```python
from build123d import *

# Parameters (mm, degrees)
SKETCH1_W           = 10
SKETCH1_H           = 10
BOSS_EXTRUDE1_DEPTH = 205
SKETCH2_R           = 3.5
BOSS_EXTRUDE2_DEPTH = 8
SKETCH4_W           = 10
SKETCH4_H           = 10
CUT_EXTRUDE1_DEPTH  = 100


with BuildPart() as part:
    # Sketch1 → Boss-Extrude1 (new body)
    with BuildSketch(Plane.XY):
        with Locations((5, -5)):
            Rectangle(SKETCH1_W, SKETCH1_H)
    extrude(amount=BOSS_EXTRUDE1_DEPTH)

    # Sketch2 → Boss-Extrude2 (add)
    with BuildSketch(Plane(origin=(10, 0, 0), x_dir=(0, 0, -1), z_dir=(1, 0, 0))):
        with Locations((-200, -5.053950804)):
            Circle(SKETCH2_R)
    extrude(amount=BOSS_EXTRUDE2_DEPTH)

    # Sketch4 → Cut-Extrude1 (cut)
    with BuildSketch(Plane(origin=(0, 0, 0), x_dir=(-1, 0, 0), z_dir=(0, 0, -1))):
        with Locations((-5, -5)):
            Rectangle(SKETCH4_W, SKETCH4_H)
    extrude(amount=-CUT_EXTRUDE1_DEPTH, mode=Mode.SUBTRACT)


solid = part.part
```
For this review, take the finished solid that the model builds, in its own axes (mm). A direction names the side the tool comes from. Coordinates: 2 decimals unless noted, no trailing zeros. Write each loop counter-clockwise with the first axis right and the second up, starting at its lowest first coordinate (ties: lowest second). Pieces come first, ordered by that corner, then holes.
(1) For pin 1 Ø2 at (x, y) = (15, -4) entering from -Z; pin 2 Ø2 at (x, y) = (10.5, -7.5) entering from +Z; pin 3 Ø10 at (x, z) = (15.5, 158) entering from -Y, all flat-tipped, find the tip position at first contact; note any pin that passes through.
(2) Tool access review of faces 1 (the face through (18, -5, 200)), 2 (the face through (13.944, -4.003, 196.662)): name each direction out of +Z, -Z, +X, -X, +Y, -Y from which nothing blocks a thin tool from reaching the whole face with its end or side.
(3) Add section B-B on y = -7. Give the boundary of the cut face in (x, z), then the cut area to 3 significant figures.
(4) Wall thickness on probe 1 along X at (y, z) = (-1, 178); probe 2 along Z at (x, y) = (10.25, -5.25); probe 3 along Z at (x, y) = (11.25, -6.25): over which ranges is each line inside the solid? List them lowest first.
(5) Add section C-C on z = 187.5. Give the boundary of the cut face in (x, y), then the cut area to 3 significant figures.
(6) Add section A-A on z = 200. Give the boundary of the cut face in (x, y).
Answer sheet:
1. pin 1: stops at z = 196.5
1. pin 2: stops at z = 205
1. pin 3: passes through
2. face 1: +Z, -Z, +X, +Y, -Y
2. face 2: +X
3. outline: (0, 100) - (10, 100) - (10, 197.09) - (18, 197.09) - (18, 202.91) - (10, 202.91) - (10, 205) - (0, 205) - close
3. area: 1,100 mm2
4. probe 1: x = 0 to 10
4. probe 2: z = 196.51 to 203.49
4. probe 3: z = 196.71 to 203.29
5. outline: (0, -10) - (10, -10) - (10, 0) - (0, 0) - close
5. area: 100 mm2
6. outline: (0, -10) - (10, -10) - (10, -8.55) - (18, -8.55) - (18, -1.55) - (10, -1.55) - (10, 0) - (0, 0) - close
